Job drawing, mm, ordinate dimensions from the low corner. One solid piece. A direction names the side the tool comes from. Round coordinates to 2 decimals unless told otherwise and drop trailing zeros. Loops run counter-clockwise (first coordinate to the right, second up) from the corner with the lowest first, then second, coordinate; pieces in that order, holes last.
1) Drop flat-ended pins along their axis: P1, Ø3, axis at y = 7, z = 2, coming from the -X side; P2, Ø1.8, axis at x = 2.5, z = 3.5, coming from the +Y side; P3, Ø1.5, axis at y = 6, z = 2.5, coming from the +X side. Give the stop position or say it passes through.
2) Probe line 1 (X direction, y = 3.75, z = 4.25); line 2 (Y direction, x = 23.75, z = 2.75). List the from-to ranges inside material, lowest first.
3) 3-axis set-ups, long thin cutter, end or side, ignore diameter. For the marked faces 1, 2, 3, 4 and 5: which of +Z, -Z, +X, -X, +Y, -Y reach the whole face in a straight line?
4) Mould opens along Z. For the marked faces 6, 7 and 8 say: +Z half, -Z half, draft (parallel to the pull), parting line (faces both ways), or undercut.
5) Band-saw the part on C-C, the plane y = 8.5. Write the cut outline in (x, z), then the cut area to 3 significant figures.
6) Band-saw the part on B-B, the plane y = 1. Write the cut outline in (x, z) (3 decimals), then the cut area to 3 significant figures.
7) Band-saw the part on D-D, the plane x = 2.75. Write the cut outline in (y, z), then the cut area to 3 significant figures.
8) Band-saw the part on A-A, the plane z = 3. Write the cut outline in (x, y).
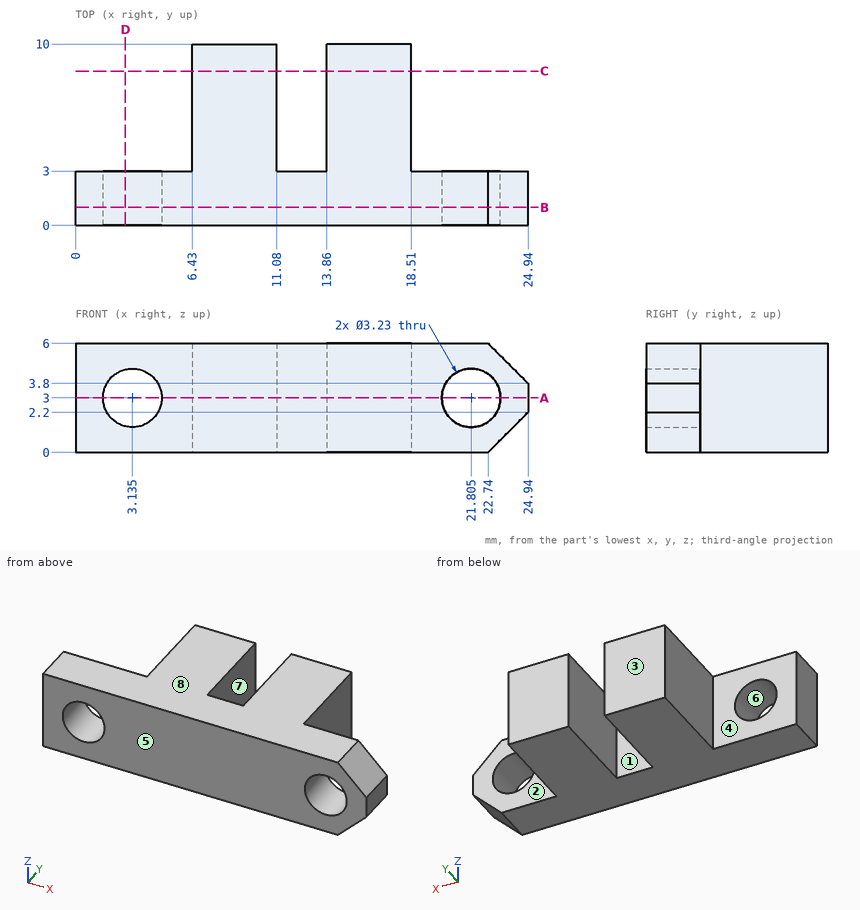
Reported:
1. P1: stops at x = 6.43
1. P2: stops at y = 3
1. P3: stops at x = 18.51
2. line 1: x = 6.43 to 11.08, 13.86 to 18.51
2. line 2: y = 0 to 3
3. face 1: +Z, -Z, +Y
3. face 2: +Z, -Z, +X, +Y
3. face 3: +Z, -Z, +X, -X, +Y
3. face 4: +Z, -Z, -X, +Y
3. face 5: +Z, -Z, +X, -X, -Y
4. face 6: undercut
4. face 7: draft
4. face 8: +Z half
5. outline: (6.43, 0) - (11.08, 0) - (11.08, 6) - (6.43, 6) - close; (13.86, 0) - (18.51, 0) - (18.51, 6) - (13.86, 6) - close
5. area: 55.8 mm2
6. outline: (0, 0) - (22.74, 0) - (24.94, 2.2) - (24.94, 3.8) - (22.74, 6) - (0, 6) - close; hole circle Ø3.23 at (3.135, 3); hole circle Ø3.23 at (21.805, 3)
6. area: 128 mm2
7. outline: (0, 0) - (3, 0) - (3, 1.43) - (0, 1.43) - close; (0, 4.57) - (3, 4.57) - (3, 6) - (0, 6) - close
7. area: 8.59 mm2
8. outline: (0, 0) - (1.52, 0) - (1.52, 3) - (0, 3) - close; (4.75, 0) - (20.19, 0) - (20.19, 3) - (18.51, 3) - (18.51, 10) - (13.86, 10) - (13.86, 3) - (11.08, 3) - (11.08, 10) - (6.43, 10) - (6.43, 3) - (4.75, 3) - close; (23.42, 0) - (24.94, 0) - (24.94, 3) - (23.42, 3) - close
